```python
from build123d import *
from build123d.topology import SkipClean

# Parameters (mm, degrees)
SKETCH1_R           = 4.25
SKETCH1_W           = 20
SKETCH1_H           = 5
BOSS_EXTRUDE1_DEPTH = 3
SKETCH2_R           = 7
SKETCH2_R_2         = 4.25
BOSS_EXTRUDE2_DEPTH = 1
FILLET1_R           = 1
CUT_EXTRUDE1_DEPTH  = 48.11952886
BOSS_EXTRUDE3_DEPTH = 16.2
BOSS_EXTRUDE3_DRAFT = 19
SKETCH5_R           = 4.25
CUT_EXTRUDE2_DEPTH  = 58.252151387


with BuildPart() as part:
    # Sketch1 → Boss-Extrude1 (new body)
    with BuildSketch(Plane.XY):
        with BuildLine():
            Line((9, -33.5), (-26, -33.5))
            ThreePointArc((-26, -33.5), (-33, -26.5), (-26, -19.5))
            Line((-26, -19.5), (-20, -19.5))
            ThreePointArc((-20, -19.5), (-16.464466094, -18.035533906), (-15, -14.5))
            Line((-15, -14.5), (-15, 28.5))
            ThreePointArc((-15, 28.5), (-13.535533906, 32.035533906), (-10, 33.5))
            Line((-10, 33.5), (10, 33.5))
            ThreePointArc((10, 33.5), (13.535533906, 32.035533906), (15, 28.5))
            Line((15, 28.5), (15, -22.894448725))
            ThreePointArc((15, -22.894448725), (15.092571663, -29.946820352), (9, -33.5))
        make_face()
        with Locations((9, -26.5)):
            Circle(SKETCH1_R, mode=Mode.SUBTRACT)
        with Locations((-26, -26.5)):
            Circle(SKETCH1_R, mode=Mode.SUBTRACT)
        with Locations((0, 26)):
            Rectangle(SKETCH1_W, SKETCH1_H, mode=Mode.SUBTRACT)
    extrude(amount=BOSS_EXTRUDE1_DEPTH)

    # Sketch2 → Boss-Extrude2 (add)
    # profile 1 of 2: a face of its own
    with BuildSketch(Plane.XY.offset(3)):
        with Locations(Location((-26, -26.5, 0), (0, 0, 270))):
            Circle(SKETCH2_R)
        with Locations((-26, -26.5)):
            Circle(SKETCH2_R_2, mode=Mode.SUBTRACT)
    # profile 2 of 2: a face of its own
    with BuildSketch(Plane.XY.offset(3)):
        with Locations(Location((9, -26.5, 0), (0, 0, 270))):
            Circle(SKETCH2_R)
        with Locations((9, -26.5)):
            Circle(SKETCH2_R_2, mode=Mode.SUBTRACT)
    extrude(amount=BOSS_EXTRUDE2_DEPTH)

    # Fillet1
    fillet1_edges = [part.edges().sort_by_distance(p)[0] for p in [
        (-26, -19.5, 4),
        (9, -19.5, 4),
    ]]
    fillet(fillet1_edges, radius=FILLET1_R - 0.0001)  # a hair under: the kernel refuses the full size

    # Sketch3 → Cut-Extrude1 (cut, through all)
    with SkipClean():  # the faces are left unmerged after this step: merging them gives an invalid solid
        with BuildSketch(Plane.XY.offset(3)):
            with BuildLine():
                Line((-20, -19.5), (9, -19.5))
                ThreePointArc((9, -19.5), (12.446820352, -20.407428337), (15, -22.894448725))
                Line((15, -22.894448725), (15, 33.5))
                Line((15, 33.5), (-20, 33.5))
                Line((-20, 33.5), (-20, -19.5))
            make_face()
        extrude(amount=-CUT_EXTRUDE1_DEPTH, mode=Mode.SUBTRACT)


with BuildPart() as boss_extrude3_tool:
    # Sketch4 → Boss-Extrude3 (with draft: the straight prism first)
    with BuildSketch(Plane.XY.offset(3)):
        with BuildLine():
            ThreePointArc((-26, -19.5), (-33, -26.5), (-26, -33.5))
            Line((-26, -33.5), (9, -33.5))
            ThreePointArc((9, -33.5), (16, -26.5), (9, -19.5))
            Line((9, -19.5), (-26, -19.5))
        make_face()
    extrude(amount=-BOSS_EXTRUDE3_DEPTH)
    # Boss-Extrude3: the draft: its side faces are tilted about the plane it starts from
    boss_extrude3_sides = [boss_extrude3_tool.faces().sort_by_distance(p)[0] for p in [
        (-33, -26.5, -5.1),
        (-8.5, -33.5, -5.1),
        (16, -26.5, -5.1),
        (-8.5, -19.5, -5.1),
    ]]
    draft(boss_extrude3_sides, Plane.XY.offset(3), BOSS_EXTRUDE3_DRAFT)


with BuildPart() as part_1:
    add(part.part)

    # Boss-Extrude3: add boss_extrude3_tool
    add(boss_extrude3_tool.part)

    # Sketch5 → Cut-Extrude2 (cut, through all)
    with BuildSketch(Plane.XY.offset(3)):
        with Locations((-26, -26.5)):
            Circle(SKETCH5_R)
        with Locations((9, -26.5)):
            Circle(SKETCH5_R)
    extrude(amount=-CUT_EXTRUDE2_DEPTH, mode=Mode.SUBTRACT)


solid = part_1.part
```
Input: part model. Units: mm. Frame: model coordinates. Give positions to 0.01 mm unless a question says otherwise; leave off trailing zeros. Write each loop counter-clockwise with the first axis right and the second up, starting at its lowest first coordinate (ties: lowest second). Pieces come first, ordered by that corner, then holes. Notation, with made-up numbers: (-24.5, -17) - (-4.5, -17) arc R15 ccw to (-4.5, -2) - close; hole circle Ø7 at (1, -22.75). An arc over 180 degrees is marked (long way). Write item = value, one per line. Start each with the question number.
1. Ray query, L1, parallel to X at y = -26.5, z = 3.6; L2, parallel to X at y = -26.5, z = 3.45; L3, parallel to Y at x = -26, z = -6.5. Return the intervals inside material, ascending.
2. First-contact query: pin 1 Ø1 at (y, z) = (-24.5, 1) entering from +X; pin 2 Ø8 at (x, z) = (1, -1) entering from -Y; pin 3 Ø3 at (x, z) = (-16, -6.5) entering from -Y; pin 4 Ø5 at (x, y) = (9, -26.5) entering from +Z. Flat tips, straight axial feed; report the tip coordinate or a pass-through.
3. Section query C-C, the plane x = -3.5. Output: boundary loops of the cut face in (y, z), then the cut area to 3 significant figures.
4. Section query D-D, the plane z = -1. Output: boundary loops of the cut face in (x, y), then the cut area to 3 significant figures.
5. Section query A-A, the plane y = -26.5. Count the separate pieces of the cut face and the enclosed holes in it, then the cut area to 3 significant figures.
6. Section query B-B, the plane z = 2. Output: boundary loops of the cut face in (x, y).
Check sheet entries:
q1.L1 = -32.8 to -30.25, -21.75 to -19.2, 2.2 to 4.75, 13.25 to 15.8
q1.L2 = -32.89 to -30.25, -21.75 to -19.11, 2.11 to 4.75, 13.25 to 15.89
q1.L3 = -36.77 to -30.75, -22.25 to -16.23
q2.pin_1 = 16.64
q2.pin_2 = -36.25
q2.pin_3 = -37.29
q2.pin_4 = through
q3.outline = (-39.08, -13.2) - (-13.92, -13.2) - (-19.5, 3) - (-33.5, 3) - close
q3.area = 317 mm2
q4.outline = (-26, -34.88) - (9, -34.88) arc R8.38 ccw to (9, -18.12) - (-26, -18.12) arc R8.38 ccw to start; hole circle Ø8.5 at (-26, -26.5); hole circle Ø8.5 at (9, -26.5)
q4.area = 693 mm2
q5.separate_pieces = 3
q5.enclosed_holes = 0
q5.area = 619 mm2
q6.outline = (-26, -33.84) - (9, -33.84) arc R7.34 ccw to (9, -19.16) - (-26, -19.16) arc R7.34 ccw to start; hole circle Ø8.5 at (-26, -26.5); hole circle Ø8.5 at (9, -26.5)
